```python
from build123d import *

# Parameters (mm, degrees)
SKETCH013_W     = 210
SKETCH013_H     = 140
PAD009_DEPTH    = 24.9
SKETCH014_R     = 6
POCKET002_DEPTH = 5
POCKET002_TAPER = 48
SKETCH015_R     = 7.6
POCKET003_DEPTH = 32
PAD013_DEPTH    = 31.2
SKETCH027_R     = 2.1
HOLE005_DEPTH   = 25
HOLE005_TIPS_R  = 2.1
SKETCH030_R     = 2.75
HOLE008_DEPTH   = 44
HOLE008_TIPS_R  = 2.75
SKETCH032_W     = 165
SKETCH032_H     = 100
POCKET008_DEPTH = 13
POCKET008_TAPER = 45
SKETCH033_R     = 1.25
HOLE009_DEPTH   = 14
HOLE009_TIPS_R  = 1.25


with BuildPart() as part:
    # Sketch013 → Pad009 (new body)
    with BuildSketch(Plane.YZ.offset(55)):
        with Locations((0, -5)):
            Rectangle(SKETCH013_W, SKETCH013_H)
    extrude(amount=-PAD009_DEPTH)

    # Sketch014 → Pocket002 (cut)
    with BuildSketch(Plane.YZ.offset(30)):
        with Locations((-70, 20)):
            Circle(SKETCH014_R)
        with Locations((70, 20)):
            Circle(SKETCH014_R)
    extrude(amount=POCKET002_DEPTH, taper=POCKET002_TAPER, mode=Mode.SUBTRACT)

    # Sketch015 → Pocket003 (cut)
    with BuildSketch(Plane.YZ.offset(30)):
        Circle(SKETCH015_R)
    extrude(amount=POCKET003_DEPTH, mode=Mode.SUBTRACT)

    # Sketch023 → Pad013 (join)
    with BuildSketch(Plane.YZ.offset(31)):
        Polygon((-105, 65), (-80, 65), (-102.5, 25), (-102.5, -50), (-45, -65), (45, -65), (102.5, -50), (102.5, 20), (80, 65), (105, 65), (105, -75), (-105, -75), align=None)
    extrude(amount=-PAD013_DEPTH)

    # Sketch027 → Hole005 (cut)
    with BuildSketch(Plane.YZ.offset(-0.2)):
        with Locations((-95, -65)):
            Circle(SKETCH027_R)
        with Locations((-75, -65)):
            Circle(SKETCH027_R)
        with Locations((95, -65)):
            Circle(SKETCH027_R)
        with Locations((75, -65)):
            Circle(SKETCH027_R)
        with Locations((-87.5, 57.5)):
            Circle(SKETCH027_R)
        with Locations((87.5, 57.5)):
            Circle(SKETCH027_R)
    extrude(amount=HOLE005_DEPTH, mode=Mode.SUBTRACT)

    # Hole005 tips → Hole005 tip 1 section 0
    with BuildSketch(Plane.YZ.offset(24.8), mode=Mode.PRIVATE) as hole005_tip_1_s0:
        with Locations((-95, -65)):
            Circle(HOLE005_TIPS_R)
    loft([hole005_tip_1_s0.sketch, Vertex(26.061807, -95, -65)], mode=Mode.SUBTRACT)

    # Hole005 tips → Hole005 tip 2 section 0
    with BuildSketch(Plane.YZ.offset(24.8), mode=Mode.PRIVATE) as hole005_tip_2_s0:
        with Locations((-75, -65)):
            Circle(HOLE005_TIPS_R)
    loft([hole005_tip_2_s0.sketch, Vertex(26.061807, -75, -65)], mode=Mode.SUBTRACT)

    # Hole005 tips → Hole005 tip 3 section 0
    with BuildSketch(Plane.YZ.offset(24.8), mode=Mode.PRIVATE) as hole005_tip_3_s0:
        with Locations((95, -65)):
            Circle(HOLE005_TIPS_R)
    loft([hole005_tip_3_s0.sketch, Vertex(26.061807, 95, -65)], mode=Mode.SUBTRACT)

    # Hole005 tips → Hole005 tip 4 section 0
    with BuildSketch(Plane.YZ.offset(24.8), mode=Mode.PRIVATE) as hole005_tip_4_s0:
        with Locations((75, -65)):
            Circle(HOLE005_TIPS_R)
    loft([hole005_tip_4_s0.sketch, Vertex(26.061807, 75, -65)], mode=Mode.SUBTRACT)

    # Hole005 tips → Hole005 tip 5 section 0
    with BuildSketch(Plane.YZ.offset(24.8), mode=Mode.PRIVATE) as hole005_tip_5_s0:
        with Locations((-87.5, 57.5)):
            Circle(HOLE005_TIPS_R)
    loft([hole005_tip_5_s0.sketch, Vertex(26.061807, -87.5, 57.5)], mode=Mode.SUBTRACT)

    # Hole005 tips → Hole005 tip 6 section 0
    with BuildSketch(Plane.YZ.offset(24.8), mode=Mode.PRIVATE) as hole005_tip_6_s0:
        with Locations((87.5, 57.5)):
            Circle(HOLE005_TIPS_R)
    loft([hole005_tip_6_s0.sketch, Vertex(26.061807, 87.5, 57.5)], mode=Mode.SUBTRACT)

    # Sketch030 → Hole008 (cut)
    with BuildSketch(Plane.XY.offset(65)):
        with Locations((20, -97.5)):
            Circle(SKETCH030_R)
        with Locations((47.5, -97.5)):
            Circle(SKETCH030_R)
        with Locations((20, 97.5)):
            Circle(SKETCH030_R)
        with Locations((47.5, 97.5)):
            Circle(SKETCH030_R)
    extrude(amount=-HOLE008_DEPTH, mode=Mode.SUBTRACT)

    # Hole008 tips → Hole008 tip 1 section 0
    with BuildSketch(Plane.XY.offset(21), mode=Mode.PRIVATE) as hole008_tip_1_s0:
        with Locations((20, -97.5)):
            Circle(HOLE008_TIPS_R)
    loft([hole008_tip_1_s0.sketch, Vertex(20, -97.5, 19.347633)], mode=Mode.SUBTRACT)

    # Hole008 tips → Hole008 tip 2 section 0
    with BuildSketch(Plane.XY.offset(21), mode=Mode.PRIVATE) as hole008_tip_2_s0:
        with Locations((47.5, -97.5)):
            Circle(HOLE008_TIPS_R)
    loft([hole008_tip_2_s0.sketch, Vertex(47.5, -97.5, 19.347633)], mode=Mode.SUBTRACT)

    # Hole008 tips → Hole008 tip 3 section 0
    with BuildSketch(Plane.XY.offset(21), mode=Mode.PRIVATE) as hole008_tip_3_s0:
        with Locations((20, 97.5)):
            Circle(HOLE008_TIPS_R)
    loft([hole008_tip_3_s0.sketch, Vertex(20, 97.5, 19.347633)], mode=Mode.SUBTRACT)

    # Hole008 tips → Hole008 tip 4 section 0
    with BuildSketch(Plane.XY.offset(21), mode=Mode.PRIVATE) as hole008_tip_4_s0:
        with Locations((47.5, 97.5)):
            Circle(HOLE008_TIPS_R)
    loft([hole008_tip_4_s0.sketch, Vertex(47.5, 97.5, 19.347633)], mode=Mode.SUBTRACT)

    # Sketch032 → Pocket008 (cut)
    with BuildSketch(Plane.YZ.offset(55)):
        with Locations((32.5, 0)):
            Rectangle(SKETCH032_W, SKETCH032_H)
    extrude(amount=-POCKET008_DEPTH, taper=POCKET008_TAPER, mode=Mode.SUBTRACT)

    # Sketch033 → Hole009 (cut)
    with BuildSketch(Plane.YZ.offset(45)):
        with Locations((-17.5, 17.5)):
            Circle(SKETCH033_R)
        with Locations((17.5, 17.5)):
            Circle(SKETCH033_R)
        with Locations((-17.5, -17.5)):
            Circle(SKETCH033_R)
        with Locations((17.5, -17.5)):
            Circle(SKETCH033_R)
    extrude(amount=-HOLE009_DEPTH, mode=Mode.SUBTRACT)

    # Hole009 tips → Hole009 tip 1 section 0
    with BuildSketch(Plane.YZ.offset(31), mode=Mode.PRIVATE) as hole009_tip_1_s0:
        with Locations((-17.5, 17.5)):
            Circle(HOLE009_TIPS_R)
    loft([hole009_tip_1_s0.sketch, Vertex(30.248924, -17.5, 17.5)], mode=Mode.SUBTRACT)

    # Hole009 tips → Hole009 tip 2 section 0
    with BuildSketch(Plane.YZ.offset(31), mode=Mode.PRIVATE) as hole009_tip_2_s0:
        with Locations((17.5, 17.5)):
            Circle(HOLE009_TIPS_R)
    loft([hole009_tip_2_s0.sketch, Vertex(30.248924, 17.5, 17.5)], mode=Mode.SUBTRACT)

    # Hole009 tips → Hole009 tip 3 section 0
    with BuildSketch(Plane.YZ.offset(31), mode=Mode.PRIVATE) as hole009_tip_3_s0:
        with Locations((-17.5, -17.5)):
            Circle(HOLE009_TIPS_R)
    loft([hole009_tip_3_s0.sketch, Vertex(30.248924, -17.5, -17.5)], mode=Mode.SUBTRACT)

    # Hole009 tips → Hole009 tip 4 section 0
    with BuildSketch(Plane.YZ.offset(31), mode=Mode.PRIVATE) as hole009_tip_4_s0:
        with Locations((17.5, -17.5)):
            Circle(HOLE009_TIPS_R)
    loft([hole009_tip_4_s0.sketch, Vertex(30.248924, 17.5, -17.5)], mode=Mode.SUBTRACT)


solid = part.part
```
The model under review builds one solid part; all positions refer to its coordinate system, in mm. A direction names the side the tool comes from. Coordinates: 2 decimals unless noted, no trailing zeros. Write each loop counter-clockwise with the first axis right and the second up, starting at its lowest first coordinate (ties: lowest second). Pieces come first, ordered by that corner, then holes. Notation, with made-up numbers: (25.5, 60.25) - (59.5, 60.25) arc R7 cw to (59.5, 73.25) - close; hole circle Ø9 at (14.25, 68). An arc over 180 degrees is marked (long way). Write item = value, one per line.
(1) Consider section A-A, the plane x = 12. Give the boundary of the cut face in (y, z), then the cut area to 3 significant figures.
Result sheet:
outline = (-105, -75) - (105, -75) - (105, 65) - (80, 65) - (102.5, 20) - (102.5, -50) - (45, -65) - (-45, -65) - (-102.5, -50) - (-102.5, 25) - (-80, 65) - (-105, 65) - close; hole circle Ø4.2 at (-95, -65); hole circle Ø4.2 at (-87.5, 57.5); hole circle Ø4.2 at (-75, -65); hole circle Ø4.2 at (75, -65); hole circle Ø4.2 at (87.5, 57.5); hole circle Ø4.2 at (95, -65)
area = 4,490 mm^2
(2) For line 1 (Z direction, x = 36.75, y = 17.5); line 2 (X direction, y = 97, z = 51); line 3 (Z direction, x = 45, y = 62.5), list the stretches that pass through material, from the lowest coordinate up. Write a range as [from, to].
Result sheet:
line_1 = [-75, -18.75], [-16.25, 16.25], [18.75, 65]
line_2 = [-0.2, 17.3], [22.7, 44.8], [50.2, 55]
line_3 = [-75, -40], [40, 65]
(3) Consider section B-B, the plane y = -61. Give the boundary of the cut face in (x, z).
Result sheet:
outline = (-0.2, -75) - (55, -75) - (55, 65) - (30.1, 65) - (30.1, -60.83) - (-0.2, -60.83) - close
(4) Machinability: for faces 4 (the face through (12.12, 72.9, -64.91)), 5 (the face through (40, -1, 65)), which of the approach directions +Z, -Z, +X, -X, +Y, -Y give a long, thin tool a straight path to every point of the face, cutting with its end or side? Answer none if there is none.
Result sheet:
face_4 = -X
face_5 = +Z, +X, -X, +Y, -Y
(5) Mouldability with a two-part tool opening along X and no side actions: class faces 1 (the face through (25.86, 87.165, 57.515)), 2 (the face through (15, -1, -65)), 3 (the face through (19.642, 100.227, 49.534)) as pulls with the +X half, pulls with the -X half, needs draft (parallel to the pull), parting line crosses it, or undercut.
Result sheet:
face_1 = pulls with the -X half
face_2 = needs draft
face_3 = undercut
(6) For P1, Ø24.5, axis at y = 0, z = 0, coming from the +X side; P2, Ø15, axis at x = 15.5, y = -17.5, coming from the +Z side; P3, Ø4, axis at y = -17.5, z = -17.5, coming from the -X side, all flat-tipped, find the tip position at first contact; note any pin that passes through.
Result sheet:
P1 = 42
P2 = -65
P3 = 30.1
